The model under review builds one solid part; all positions refer to its coordinate system, in mm. Face numbers are marked on the shaded views. A direction names the side the tool comes from. Coordinates: 2 decimals unless noted, no trailing zeros. Write each loop counter-clockwise with the first axis right and the second up, starting at its lowest first coordinate (ties: lowest second). Pieces come first, ordered by that corner, then holes.
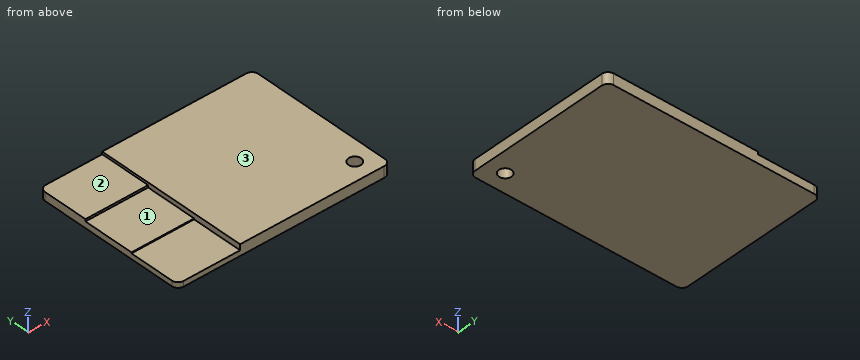
```python
from build123d import *

# Parameters (mm, degrees)
F0_W     = 68
F0_H     = 49
F1_DEPTH = 3.5
F3_DEPTH = 20
F4_R     = 2
F5_DEPTH = 3.501
F6_R     = 2


with BuildPart() as f1:
    # F0 (on Top) → F1 (new body)
    with BuildSketch(Plane.XY):
        Rectangle(F0_W, F0_H)
    extrude(amount=F1_DEPTH)

    # F2 (on face) → F3 (cut)
    with BuildSketch(Plane(origin=(-34, 0, 0), x_dir=(0, -1, 0), z_dir=(-1, 0, 0))):
        Polygon((24.5, 3.5), (-24.5, 3.5), (-24.5, 2.7), (-8.166667, 2.7), (-8.166667, 2), (8.166667, 2), (8.166667, 1.7), (24.5, 1.7), align=None)
    extrude(amount=-F3_DEPTH, mode=Mode.SUBTRACT)

    # F4 (on Top) → F5 (cut, through all)
    with BuildSketch(Plane.XY):
        with Locations((28, -18.5)):
            Circle(F4_R)
    extrude(amount=F5_DEPTH, mode=Mode.SUBTRACT)

    # F6
    f6_edges = [f1.edges().sort_by_distance(p)[0] for p in [
        (34, 24.5, 1.75),
        (34, -24.5, 1.75),
        (-34, 24.5, 1.35),
        (-34, -24.5, 0.85),
    ]]
    fillet(f6_edges, radius=F6_R)


solid = f1.part
```
Item 1: To check wall thickness, follow line 1 along Y through (x, z) = (28, 1.2); line 2 along X through (y, z) = (-18.5, 1.1); line 3 along Z through (x, y) = (-24, 19.5). State the ranges of each line that lie inside material, in increasing order.
Solved:
line 1: y = -24.5 to -20.5, -16.5 to 24.5
line 2: x = -34 to 26, 30 to 34
line 3: z = 0 to 2.7
Item 2: Take a section at A-A, the plane y = -18.5. Write out the cut boundary in (x, z).
Solved:
outline: (-34, 0) - (26, 0) - (26, 3.5) - (-14, 3.5) - (-14, 1.7) - (-34, 1.7) - close; (30, 0) - (34, 0) - (34, 3.5) - (30, 3.5) - close
Item 3: Take a section at C-C, the plane y = 21. Write out the cut boundary in (x, z), plus the area to 3 significant figures.
Solved:
outline: (-34, 0) - (34, 0) - (34, 3.5) - (-14, 3.5) - (-14, 2.7) - (-34, 2.7) - close
area: 222 mm2
Item 4: Machinability: for the marked faces 1, 2 and 3, which of the approach directions +Z, -Z, +X, -X, +Y, -Y give a long, thin tool a straight path to every point of the face, cutting with its end or side? Answer none if there is none.
Solved:
face 1: +Z, -X, -Y
face 2: +Z, -X, +Y, -Y
face 3: +Z, +X, -X, +Y, -Y
Item 5: Take a section at B-B, the plane x = 28. Write out the cut boundary in (y, z).
Solved:
outline: (-24.5, 0) - (-20.5, 0) - (-20.5, 3.5) - (-24.5, 3.5) - close; (-16.5, 0) - (24.5, 0) - (24.5, 3.5) - (-16.5, 3.5) - close
Item 6: Take a section at D-D, the plane x = -23. Write out the cut boundary in (y, z).
Solved:
outline: (-24.5, 0) - (24.5, 0) - (24.5, 2.7) - (8.17, 2.7) - (8.17, 2) - (-8.17, 2) - (-8.17, 1.7) - (-24.5, 1.7) - close
Item 7: For pin 1 (5 mm diameter, centred on x = -26.5, y = 0, fed in from +Z); pin 2 (0.9 mm diameter, centred on y = -11, z = 2.5, fed in from -X); pin 3 (13 mm diameter, centred on x = -29, y = -19.5, fed in from +Z), all flat-tipped, find the tip position at first contact; note any pin that passes through.
Solved:
pin 1: stops at z = 2
pin 2: stops at x = -14
pin 3: stops at z = 1.7
